Geometry: final body of the model. Coordinates: model frame, mm. Give positions to 0.01 mm unless a question says otherwise; leave off trailing zeros. Order: outer loops, then holes, each group sorted by start corner. A loop starts at its lowest first (then second) coordinate and runs counter-clockwise, first axis right, second up. Notation, with made-up numbers: (-25.5, -15) - (-0.5, -15) arc R17 cw to (-0.5, -2) - close; hole circle Ø2 at (67, -5.75). An arc over 180 degrees is marked (long way). Use one line per item in the form item = value.
from build123d import *

# Parameters (mm, degrees)
F0_W     = 101.6
F0_H     = 76.2
F1_DEPTH = 50.8
F2_R     = 5.08
F4_DEPTH = 25.4


with BuildPart() as f1:
    # F0 (on Top) → F1 (new body)
    with BuildSketch(Plane.XY):
        Rectangle(F0_W, F0_H)
    extrude(amount=F1_DEPTH)

    # F2
    f2_edges = [f1.edges().sort_by_distance(p)[0] for p in [
        (-50.8, -38.1, 25.4),
        (50.8, -38.1, 25.4),
        (0, -38.1, 0),
        (0, -38.1, 50.8),
        (50.8, 38.1, 25.4),
        (50.8, 0, 0),
        (50.8, 0, 50.8),
        (0, 38.1, 50.8),
        (-50.8, 0, 50.8),
        (-50.8, 38.1, 25.4),
        (0, 38.1, 0),
        (-50.8, 0, 0),
    ]]
    fillet(f2_edges, radius=F2_R)

    # F3 (on face) → F4 (join)
    with BuildSketch(Plane(origin=(0, 0, 0), x_dir=(1, 0, 0), z_dir=(0, 0, -1))):
        with BuildLine():
            Line((36.22162, -26.010673), (33.04662, -26.010673))
            ThreePointArc((33.04662, -26.010673), (36.22162, -29.185673), (39.39662, -26.010673))
            ThreePointArc((39.39662, -26.010673), (38.466684, -23.765609), (36.22162, -22.835673))
            Line((36.22162, -22.835673), (36.22162, -26.010673))
        make_face()
        with BuildLine():
            ThreePointArc((36.22162, -22.835673), (33.976556, -23.765609), (33.04662, -26.010673))
            Line((33.04662, -26.010673), (36.22162, -26.010673))
            Line((36.22162, -26.010673), (36.22162, -22.835673))
        make_face()
        with BuildLine():
            ThreePointArc((33.04662, 26.010673), (33.976556, 23.765609), (36.22162, 22.835673))
            Line((36.22162, 22.835673), (36.22162, 26.010673))
            Line((36.22162, 26.010673), (33.04662, 26.010673))
        make_face()
        with BuildLine():
            Line((36.22162, 26.010673), (36.22162, 22.835673))
            ThreePointArc((36.22162, 22.835673), (38.466684, 23.765609), (39.39662, 26.010673))
            ThreePointArc((39.39662, 26.010673), (36.22162, 29.185673), (33.04662, 26.010673))
            Line((33.04662, 26.010673), (36.22162, 26.010673))
        make_face()
        with BuildLine():
            Line((-36.22162, 26.010673), (-36.22162, 22.835673))
            ThreePointArc((-36.22162, 22.835673), (-33.976556, 23.765609), (-33.04662, 26.010673))
            Line((-33.04662, 26.010673), (-36.22162, 26.010673))
        make_face()
        with BuildLine():
            ThreePointArc((-33.04662, 26.010673), (-38.466684, 28.255738), (-36.22162, 22.835673))
            Line((-36.22162, 22.835673), (-36.22162, 26.010673))
            Line((-36.22162, 26.010673), (-33.04662, 26.010673))
        make_face()
        with BuildLine():
            Line((-36.22162, -26.010673), (-33.04662, -26.010673))
            ThreePointArc((-33.04662, -26.010673), (-33.976556, -23.765609), (-36.22162, -22.835673))
            Line((-36.22162, -22.835673), (-36.22162, -26.010673))
        make_face()
        with BuildLine():
            ThreePointArc((-36.22162, -22.835673), (-38.466684, -28.255738), (-33.04662, -26.010673))
            Line((-33.04662, -26.010673), (-36.22162, -26.010673))
            Line((-36.22162, -26.010673), (-36.22162, -22.835673))
        make_face()
    extrude(amount=F4_DEPTH)


solid = f1.part
(1) Cut plane C-C on y = -16.5. Output: boundary loops of the cut face in (x, z), plus the area to 3 significant figures.
Computed values:
outline = (-50.8, 5.08) arc R5.08 ccw to (-45.72, 0) - (45.72, 0) arc R5.08 ccw to (50.8, 5.08) - (50.8, 45.72) arc R5.08 ccw to (45.72, 50.8) - (-45.72, 50.8) arc R5.08 ccw to (-50.8, 45.72) - close
area = 5,140 mm²
(2) Cut plane A-A on z = -4. Output: boundary loops of the cut face in (x, y) (3 decimals).
Computed values:
outline = circle Ø6.35 at (-36.222, -26.011); circle Ø6.35 at (-36.222, 26.011); circle Ø6.35 at (36.222, -26.011); circle Ø6.35 at (36.222, 26.011)
(3) Contact query for a flat-ended pin moving along its axis: pin 1 Ø3 at (x, y) = (0.5, -12.5) entering from -Z. Output: stop coordinate, or through.
Computed values:
pin_1 = 0
(4) Ray query, line 1 along Z through (x, y) = (43, -31); line 2 along Y through (x, z) = (-9.5, 5); line 3 along Y through (x, z) = (-42.5, 1.5). Return the intervals inside material, ascending.
Computed values:
line_1 = 0 to 50.8
line_2 = -38.1 to 38.1
line_3 = -36.62 to 36.62
(5) Cut plane B-B on x = 43.5. Output: boundary loops of the cut face in (y, z), plus the area to 3 significant figures.
Computed values:
outline = (-38.1, 5.08) arc R5.08 ccw to (-33.02, 0) - (33.02, 0) arc R5.08 ccw to (38.1, 5.08) - (38.1, 45.72) arc R5.08 ccw to (33.02, 50.8) - (-33.02, 50.8) arc R5.08 ccw to (-38.1, 45.72) - close
area = 3,850 mm²
